Here's how the part is built. I have some questions about the finished solid (model axes, mm). Face numbers are marked on the shaded views. A direction names the side the tool comes from. Coordinates: 2 decimals unless noted, no trailing zeros. Loops run counter-clockwise (first coordinate to the right, second up) from the corner with the lowest first, then second, coordinate; pieces in that order, holes last. Notation, with made-up numbers: M 14,35 L 70,35 A28 ccw 70,54 Z; hole C 24.5,-38.75 d8. An arc over 180 degrees is marked long. Use one line per item in the form item = value. Start each with the question number.
(1) Imagine slicing it at B-B, the plane y = 0. Please give me the cut outline in (x, z).
(2) Imagine slicing it at C-C, the plane z = 11.5. Please give me the cut outline in (x, y).
(3) Imagine slicing it at A-A, the plane x = 0. Please give me the cut outline in (y, z).
(4) Imagine slicing it at D-D, the plane x = 8.75. Please give me the cut outline in (y, z).
(5) Thinking about a two-plate mould opening in Y: for the marked faces 3, 4 and 5, which applies, +Y half, -Y half, draft (parallel to the pull), parting line (faces both ways), or undercut?
(6) On a 3-axis mill with a long thin cutter (end or side, diameter ignored), from which of +Z, -Z, +X, -X, +Y, -Y can I reach the whole of each face in a straight line? I mean the marked faces 1 and 2. Say none if no direction works.
(7) Will these pins go through, and if not, where does the flat tip stop? P1, Ø5, axis at y = -3.5, z = 1.5, coming from the +X side; P2, Ø0.7, axis at y = 8, z = 5.5, coming from the +X side; P3, Ø3, axis at y = 8, z = 5, coming from the -X side.
(8) Please list where these lines run through material, in increasing order: L1, parallel to Y at x = 0, z = 5.5; L2, parallel to Y at x = -5, z = 4.25; L3, parallel to X at y = 1, z = 4.75.
```python
from build123d import *

# Parameters (mm, degrees)
SKETCH1_R           = 10.4
SKETCH1_R_2         = 7.8
BOSS_EXTRUDE1_DEPTH = 15
CUT_EXTRUDE1_REACH  = 17
SKETCH2_W           = 2.8
SKETCH2_H           = 2.8


with BuildPart() as part:
    # Sketch1 → Boss-Extrude1 (new body)
    with BuildSketch(Plane.XY):
        Circle(SKETCH1_R)
        Circle(SKETCH1_R_2, mode=Mode.SUBTRACT)
    extrude(amount=BOSS_EXTRUDE1_DEPTH)

    # Sketch2 → Cut-Extrude1 (cut, up to next)
    with BuildSketch(Plane.XY.offset(15), mode=Mode.PRIVATE) as cut_extrude1_sk1:
        with Locations((0, 7.1)):
            Rectangle(SKETCH2_W, SKETCH2_H)
    cut_extrude1_tool1 = extrude(cut_extrude1_sk1.sketch, amount=-CUT_EXTRUDE1_REACH, mode=Mode.PRIVATE) & part.part
    add(cut_extrude1_tool1.solids().sort_by_distance((0, 7.1, 15))[0], mode=Mode.SUBTRACT)


solid = part.part
```
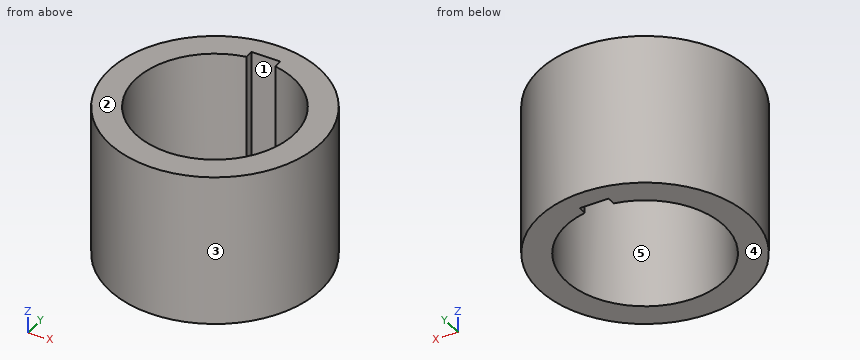
Answer:
q1.outline = M -10.4,0 L -7.8,0 L -7.8,15 L -10.4,15 Z; M 7.8,0 L 10.4,0 L 10.4,15 L 7.8,15 Z
q2.outline = C 0,0 d20.8; hole M -1.4,7.67 A7.8 ccw long 1.4,7.67 L 1.4,8.5 L -1.4,8.5 Z
q3.outline = M -10.4,0 L -7.8,0 L -7.8,15 L -10.4,15 Z; M 8.5,0 L 10.4,0 L 10.4,15 L 8.5,15 Z
q4.outline = M -5.62,0 L 5.62,0 L 5.62,15 L -5.62,15 Z
q5.face_3 = parting line
q5.face_4 = draft
q5.face_5 = undercut
q6.face_1 = +Z, -Z
q6.face_2 = +Z, +X, -X, +Y, -Y
q7.P1 = 10.35
q7.P2 = 7.05
q7.P3 = -8.12
q8.L1 = -10.4 to -7.8, 8.5 to 10.4
q8.L2 = -9.12 to -5.99, 5.99 to 9.12
q8.L3 = -10.35 to -7.74, 7.74 to 10.35
